```python
from build123d import *

# Parameters (mm, degrees)
ESQUISSE1_W                = 20
ESQUISSE1_H                = 120
EXTRUSION1_DEPTH           = 2
ESQUISSE2_R                = 1.5
EXTRUSION2_DEPTH           = 2
ESQUISSE3_R                = 1.5
EXTRUSION3_DEPTH           = 2
R_P_TITION_LIN_AIRE1_COUNT = 2
R_P_TITION_LIN_AIRE1_PITCH = 105
ESQUISSE4_R                = 1.5
ENL_V_MAT_EXTRU_1_DEPTH    = 61.860496219


with BuildPart() as part:
    # Esquisse1 → Extrusion1 (new body)
    with BuildSketch(Plane.XY):
        Rectangle(ESQUISSE1_W, ESQUISSE1_H)
    extrude(amount=EXTRUSION1_DEPTH)

    # Esquisse2 → Extrusion2 (cut)
    with BuildSketch(Plane.XY.offset(2)):
        with Locations((-5, 52.5)):
            Circle(ESQUISSE2_R)
    extrusion2 = extrude(amount=-EXTRUSION2_DEPTH, mode=Mode.SUBTRACT)

    # Esquisse3 → Extrusion3 (cut)
    with BuildSketch(Plane.XY.offset(2)):
        with Locations((5, 52.5)):
            Circle(ESQUISSE3_R)
    extrusion3 = extrude(amount=-EXTRUSION3_DEPTH, mode=Mode.SUBTRACT)

    # Répétition linéaire1: Extrusion2, Extrusion3 ×2
    with Locations(*[(0, -i * R_P_TITION_LIN_AIRE1_PITCH, 0) for i in range(1, R_P_TITION_LIN_AIRE1_COUNT)]):
        add(extrusion2, mode=Mode.SUBTRACT)
        add(extrusion3, mode=Mode.SUBTRACT)

    # Esquisse4 → Enlèv. mat.-Extru.1 (cut, through all)
    with BuildSketch(Plane(origin=(0, 0, 0), x_dir=(-1, 0, 0), z_dir=(0, 0, -1))):
        with Locations((-5, 40)):
            Circle(ESQUISSE4_R)
        with Locations((5, 30)):
            Circle(ESQUISSE4_R)
    extrude(amount=-ENL_V_MAT_EXTRU_1_DEPTH, mode=Mode.SUBTRACT)


solid = part.part
```
Source: CAD feature listing. Evaluate the final solid. Frame: model axes, mm. Round coordinates to 2 decimals unless told otherwise and drop trailing zeros. Loops run counter-clockwise (first coordinate to the right, second up) from the corner with the lowest first, then second, coordinate; pieces in that order, holes last.
1. Ray query, L1, parallel to Y at x = 5, z = 1.6; L2, parallel to Y at x = 6, z = 1.8; L3, parallel to X at y = 41, z = 1.1. Return the intervals inside material, ascending.
2. Section query C-C on y = 30. Output: boundary loops of the cut face in (x, z).
3. Section query B-B on x = 5. Output: boundary loops of the cut face in (y, z), and give its area (3 significant figures).
4. Section query D-D on z = 0.35. Output: boundary loops of the cut face in (x, y).
5. Section query A-A on y = -52.5. Output: boundary loops of the cut face in (x, z).
6. Mould query, pull axis Y, two halves, no side actions, for faces 1 (the cylindrical face through (-5, 51, 1)), 2 (the flat face through (0, 60, 1)), 3 (the flat face through (0, 1, 2)). Classes: released by +Y, released by -Y, zero draft, split by the parting line, or undercut.
Answers below:
1. L1: y = -60 to -54, -51 to 38.5, 41.5 to 51, 54 to 60
1. L2: y = -60 to -53.62, -51.38 to 38.88, 41.12 to 51.38, 53.62 to 60
1. L3: x = -10 to 3.88, 6.12 to 10
2. outline: (-10, 0) - (-6.5, 0) - (-6.5, 2) - (-10, 2) - close; (-3.5, 0) - (10, 0) - (10, 2) - (-3.5, 2) - close
3. outline: (-60, 0) - (-54, 0) - (-54, 2) - (-60, 2) - close; (-51, 0) - (38.5, 0) - (38.5, 2) - (-51, 2) - close; (41.5, 0) - (51, 0) - (51, 2) - (41.5, 2) - close; (54, 0) - (60, 0) - (60, 2) - (54, 2) - close
3. area: 222 mm2
4. outline: (-10, -60) - (10, -60) - (10, 60) - (-10, 60) - close; hole circle Ø3 at (-5, -52.5); hole circle Ø3 at (-5, 30); hole circle Ø3 at (-5, 52.5); hole circle Ø3 at (5, -52.5); hole circle Ø3 at (5, 40); hole circle Ø3 at (5, 52.5)
5. outline: (-10, 0) - (-6.5, 0) - (-6.5, 2) - (-10, 2) - close; (-3.5, 0) - (3.5, 0) - (3.5, 2) - (-3.5, 2) - close; (6.5, 0) - (10, 0) - (10, 2) - (6.5, 2) - close
6. face 1: undercut
6. face 2: released by +Y
6. face 3: zero draft
